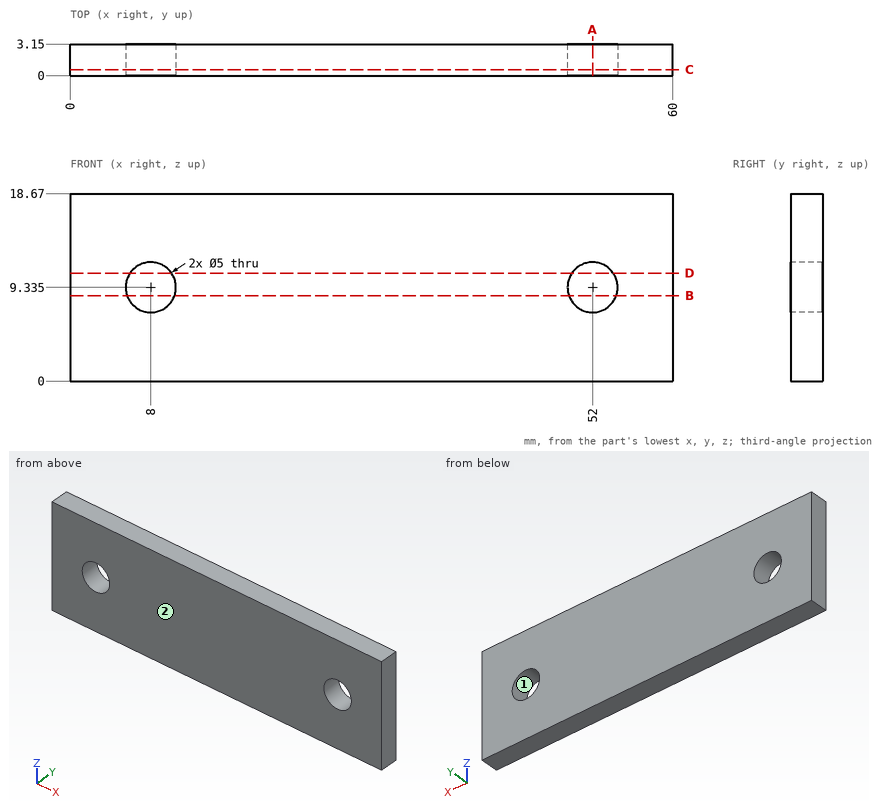
Part print with two shaded views. Sizes in mm from the minimum x, y, z corner. Round coordinates to 2 decimals unless told otherwise and drop trailing zeros. Order: outer loops, then holes, each group sorted by start corner. A loop starts at its lowest first (then second) coordinate and runs counter-clockwise, first axis right, second up. Notation, with made-up numbers: (25, 52.25) -> (84, 52.25) arc R12 cw to (84, 61.25) -> close; hole circle Ø6 at (62, 8). An arc over 180 degrees is marked (long way). Write each question's results on one line, items separated by ' | '.
1. Pull direction X, two halves, no side cores. Call the marked faces 1 and 2: pulls with the +X half, pulls with the -X half, needs draft (parallel to the pull), parting line crosses it, or undercut.
Findings below:
face 1: undercut | face 2: needs draft
2. Cut at B-B (z = 8.5). Give the cut face in (x, y), plus the area to 3 significant figures.
Findings below:
outline: (0, 0) -> (5.64, 0) -> (5.64, 3.15) -> (0, 3.15) -> close; (10.36, 0) -> (49.64, 0) -> (49.64, 3.15) -> (10.36, 3.15) -> close; (54.36, 0) -> (60, 0) -> (60, 3.15) -> (54.36, 3.15) -> close | area: 159 mm²
3. Cut at D-D (z = 10.75). Give the cut face in (x, y).
Findings below:
outline: (0, 0) -> (5.94, 0) -> (5.94, 3.15) -> (0, 3.15) -> close; (10.06, 0) -> (49.94, 0) -> (49.94, 3.15) -> (10.06, 3.15) -> close; (54.06, 0) -> (60, 0) -> (60, 3.15) -> (54.06, 3.15) -> close
4. Cut at C-C (y = 0.6). Give the cut face in (x, z) (3 decimals), plus the area to 3 significant figures.
Findings below:
outline: (0, 0) -> (60, 0) -> (60, 18.67) -> (0, 18.67) -> close; hole circle Ø5 at (8, 9.335); hole circle Ø5 at (52, 9.335) | area: 1,080 mm²
5. Cut at A-A (x = 52). Give the cut face in (y, z) (3 decimals).
Findings below:
outline: (0, 0) -> (3.15, 0) -> (3.15, 6.835) -> (0, 6.835) -> close; (0, 11.835) -> (3.15, 11.835) -> (3.15, 18.67) -> (0, 18.67) -> close
6. Wall check: line 1 along X through (y, z) = (2.7, 11); line 2 along Z through (x, y) = (52, 2.2) (3 decimals); line 3 along X through (y, z) = (2.15, 9.75). Give the ranges that are in metal, low to high. Write a range as [from, to].
Findings below:
line 1: x = [0, 6.14], [9.86, 50.14], [53.86, 60] | line 2: z = [0, 6.835], [11.835, 18.67] | line 3: x = [0, 5.53], [10.47, 49.53], [54.47, 60]
